The figure shows three views and two pictorial views of one solid part (mm, origin at its lowest corner). Answer the questions. Coordinates: 2 decimals unless noted, no trailing zeros. Order: outer loops, then holes, each group sorted by start corner. A loop starts at its lowest first (then second) coordinate and runs counter-clockwise, first axis right, second up.
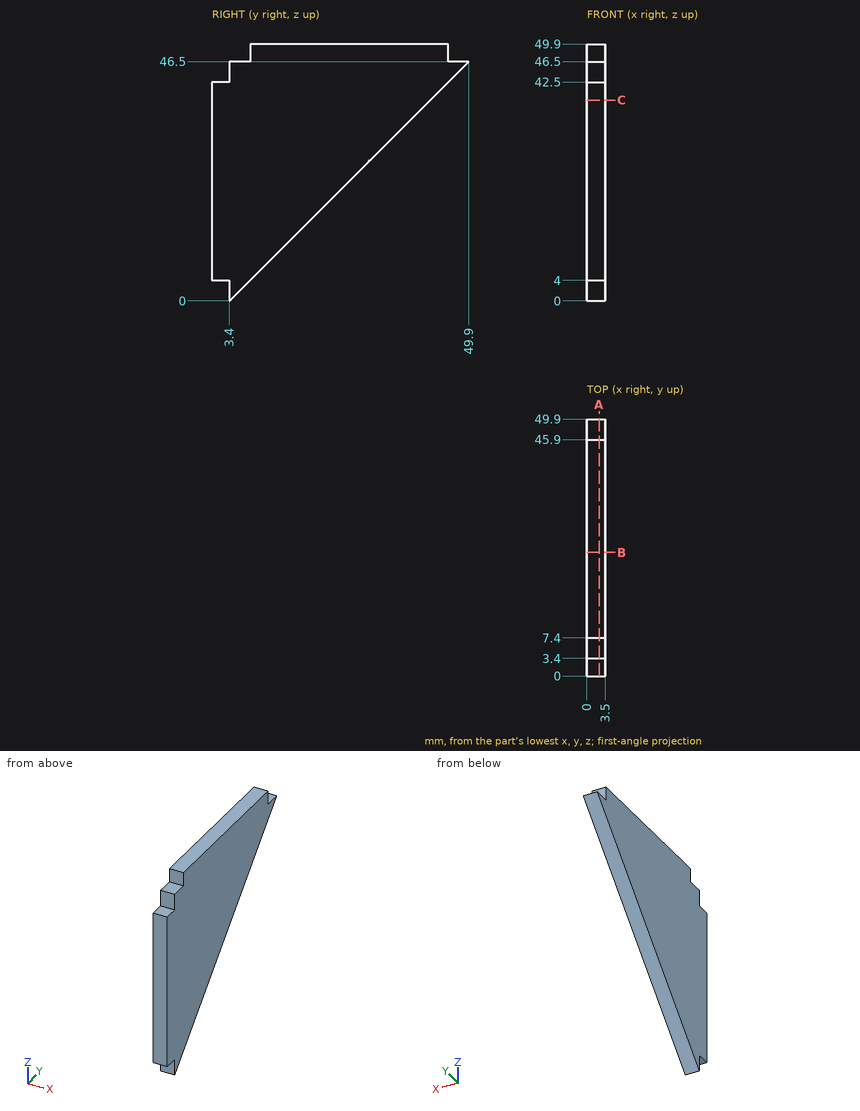
1) Straight lines are drawn through the part: probe 1 along Y at (x, z) = (2.9, 47); probe 2 along Y at (x, z) = (0.9, 12.5); probe 3 along Z at (x, y) = (1.9, 45). For each, find the intervals that lie inside material, in ascending order.
2) A cutting plane is placed at C-C, the plane z = 39. Write down the section's boundary in (x, y).
3) A cutting plane is placed at A-A, the plane x = 2.35. Write down the section's boundary in (y, z), plus the area to 3 significant figures.
4) Each of these flat-tipped pins is pushed along its axis until it touches: P1, Ø2, axis at x = 3, y = 43, coming from the -Z side; P2, Ø1, axis at x = 2, y = 5.5, coming from the +Z side; P3, Ø4, axis at y = 25.5, z = 23, coming from the -X side; P4, Ø1.8, axis at x = 2.5, z = 45, coming from the -Y side. Where does it stop, or does it pass through?
5) A cutting plane is placed at B-B, the plane y = 24. Write down the section's boundary in (x, z).
Working result:
1. probe 1: y = 7.4 to 45.9
1. probe 2: y = 0 to 15.9
1. probe 3: z = 41.6 to 49.9
2. outline: (0, 0) - (3.5, 0) - (3.5, 42.4) - (0, 42.4) - close
3. outline: (0, 4) - (3.4, 4) - (3.4, 0) - (49.9, 46.5) - (45.9, 46.5) - (45.9, 49.9) - (7.4, 49.9) - (7.4, 46.5) - (3.4, 46.5) - (3.4, 42.5) - (0, 42.5) - close
3. area: 1,340 mm2
4. P1: stops at z = 38.6
4. P2: stops at z = 46.5
4. P3: stops at x = 0
4. P4: stops at y = 3.4
5. outline: (0, 20.6) - (3.5, 20.6) - (3.5, 49.9) - (0, 49.9) - close
